Design review of the part built by this model. Coordinates are the model's own, in mm. A direction names the side the tool comes from. Coordinates: 2 decimals unless noted, no trailing zeros. Loops run counter-clockwise (first coordinate to the right, second up) from the corner with the lowest first, then second, coordinate; pieces in that order, holes last. Notation, with made-up numbers: (62.25, 16) -> (75.25, 16) arc R26 cw to (75.25, 38) -> close; hole circle Ø3 at (-30.5, 47.5). An arc over 180 degrees is marked (long way). Use a Markdown table: item, result. Add a question column.
Q1. Take a section at B-B on y = 7. Write out the cut boundary in (x, z).
Q2. Take a section at A-A on x = 4.25. Write out the cut boundary in (y, z), plus the area to 3 significant figures.
Q3. For probe 1 along Y at (x, z) = (-3.75, 3); probe 2 along Y at (x, z) = (3.5, 0); probe 3 along X at (y, z) = (9.5, -3), list the stretches that pass through material, from the lowest coordinate up.
Q4. Draft analysis for pull direction Y (two halves, no side actions). For faces 1 (the face through (5, 1, 0)), 2 (the face through (3, 10, 0)), 3 (the face through (-3, 10.5, 0)), state which applies: pulls with the +Y half, pulls with the -Y half, needs draft (parallel to the pull), parting line crosses it, or undercut.
Q5. Clearance check with flat-ended pins moving along their axes: pin 1 Ø1.5 at (y, z) = (6, -1) entering from -X; pin 2 Ø4 at (y, z) = (2, 3.5) entering from -X; pin 3 Ø1.2 at (y, z) = (9, -0.5) entering from -X. State where each tip first meets the part, or that it passes through.
Q6. For faces 4 (the face through (-2, 7.6, -0.1)), 5 (the face through (3, 10.5, 0)), 6 (the face through (0.867, 2.514, 3.905)), list the 3-axis set-ups (+Z, -Z, +X, -X, +Y, -Y) from which the entire face can be reached by the end or side of a thin tool; tool diameter is ignored.
Q7. Take a section at D-D on z = -2. Write out the cut boundary in (x, y).
Q8. Take a section at C-C on x = 0. Write out the cut boundary in (y, z).
from build123d import *

# Parameters (mm, degrees)
CUT_EXTRUDE1_DEPTH    = 4
F_2_0MM_DOWEL_HOLE1_D = 2


with BuildPart() as part:
    # Sketch2 → Revolve1 (revolve)
    with BuildSketch(Plane.XY, mode=Mode.PRIVATE) as revolve1_sk:
        Polygon((0, 0), (5, 0), (5, 1.5), (4, 1.5), (4, 3.5), (5, 3.5), (5, 10.5), (0, 10.5), align=None)
    revolve(revolve1_sk.sketch.rotate(Axis((0, 10.5, 0), (0, -1, 0)), 180), axis=Axis((0, 10.5, 0), (0, -1, 0)))

    # Sketch3 → Cut-Extrude1 (cut)
    with BuildSketch(Plane(origin=(0, 10.5, 0), x_dir=(1, 0, 0), z_dir=(0, 1, 0))):
        with BuildLine():
            Line((-2, 4.582575695), (-2, -4.582575695))
            ThreePointArc((-2, -4.582575695), (0, -5), (2, -4.582575695))
            Line((2, -4.582575695), (2, 4.582575695))
            ThreePointArc((2, 4.582575695), (0, 5), (-2, 4.582575695))
        make_face()
    extrude(amount=-CUT_EXTRUDE1_DEPTH, mode=Mode.SUBTRACT)

    # Ø2.0mm Dowel Hole1 (through all)
    with Locations(Plane(origin=(5, 0, 0), x_dir=(0, 0, -1), z_dir=(1, 0, 0))):
        with Locations((0, 9)):
            Hole(F_2_0MM_DOWEL_HOLE1_D / 2)


solid = part.part
Answer list:
| question | item | result |
|---|---|---|
| 1 | outline | (-2, -4.58) -> (-2, 4.58) arc R5 ccw to start; (2, -4.58) arc R5 ccw to (2, 4.58) -> close |
| 2 | outline | (0, -2.63) -> (1.5, -2.63) -> (1.5, 2.63) -> (0, 2.63) -> close; (3.5, -2.63) -> (10.5, -2.63) -> (10.5, 2.63) -> (3.5, 2.63) -> close; hole circle Ø2 at (9, 0) |
| 2 | area | 41.6 mm² |
| 3 | probe 1 | 0 to 1.5, 3.5 to 10.5 |
| 3 | probe 2 | 0 to 8, 10 to 10.5 |
| 3 | probe 3 | -4 to -2, 2 to 4 |
| 4 | face 1 | needs draft |
| 4 | face 2 | undercut |
| 4 | face 3 | pulls with the +Y half |
| 5 | pin 1 | x = -4.99 |
| 5 | pin 2 | x = -4.75 |
| 5 | pin 3 | x = -4.92 |
| 6 | face 4 | +Z, -Z, +Y |
| 6 | face 5 | +Z, -Z, +X, -X, +Y |
| 6 | face 6 | none |
| 7 | outline | (-4.58, 0) -> (4.58, 0) -> (4.58, 1.5) -> (3.46, 1.5) -> (3.46, 3.5) -> (4.58, 3.5) -> (4.58, 10.5) -> (2, 10.5) -> (2, 6.5) -> (-2, 6.5) -> (-2, 10.5) -> (-4.58, 10.5) -> (-4.58, 3.5) -> (-3.46, 3.5) -> (-3.46, 1.5) -> (-4.58, 1.5) -> close |
| 8 | outline | (0, -5) -> (1.5, -5) -> (1.5, -4) -> (3.5, -4) -> (3.5, -5) -> (6.5, -5) -> (6.5, 5) -> (3.5, 5) -> (3.5, 4) -> (1.5, 4) -> (1.5, 5) -> (0, 5) -> close |
